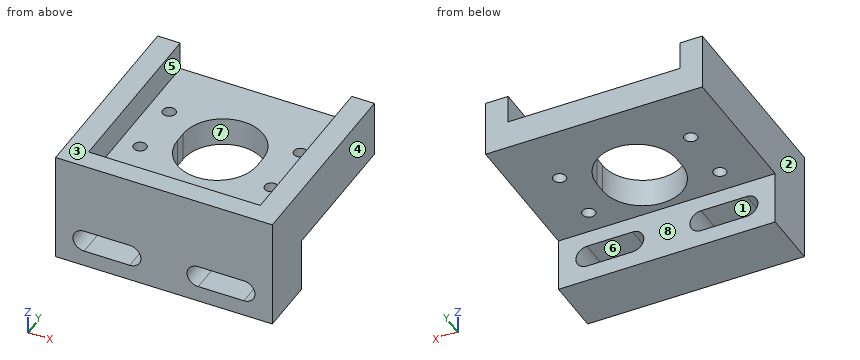
from build123d import *

# Parameters (mm, degrees)
SKETCH1_W                = 38
SKETCH1_H                = 19.5
BOSS_EXTRUDE1_DEPTH      = 35
SKETCH2_W                = 38
SKETCH2_H                = 9.5
CUT_EXTRUDE1_DEPTH       = 25
F_6_32_SLOT_REACH        = 12
APERTURE_THRU_HOLE_REACH = 21.5
SKETCH5_4_R              = 1.13
CUT_EXTRUDE5_DEPTH       = 5
F_4_40_TAPPED_HOLE1_D    = 2.2606


with BuildPart() as part:
    # Sketch1 → Boss-Extrude1 (new body)
    with BuildSketch(Plane(origin=(0, 0, 0), x_dir=(1, 0, 0), z_dir=(0, 1, 0))):
        with Locations((-7.223776224, 34.305944056)):
            Rectangle(SKETCH1_W, SKETCH1_H)
    extrude(amount=BOSS_EXTRUDE1_DEPTH)

    # Sketch2 → Cut-Extrude1 (cut)
    with BuildSketch(Plane(origin=(0, 35, 0), x_dir=(1, 0, 0), z_dir=(0, 1, 0))):
        with Locations((-7.223776224, 39.305944056)):
            Rectangle(SKETCH2_W, SKETCH2_H)
    extrude(amount=-CUT_EXTRUDE1_DEPTH, mode=Mode.SUBTRACT)

    # Sketch4 → 6-32 slot (cut, up to next)
    with BuildSketch(Plane(origin=(0, 10, 0), x_dir=(1, 0, 0), z_dir=(0, 1, 0)), mode=Mode.PRIVATE) as f_6_32_slot_sk1:
        with BuildLine():
            ThreePointArc((-13.223776224, 41.225951608), (-11.268776224, 39.270951608), (-13.223776224, 37.315951608))
            Line((-13.223776224, 37.315951608), (-21.223776224, 37.315951608))
            ThreePointArc((-21.223776224, 37.315951608), (-23.178776224, 39.270951608), (-21.223776224, 41.225951608))
            Line((-21.223776224, 41.225951608), (-13.223776224, 41.225951608))
        make_face()
    f_6_32_slot_tool1 = extrude(f_6_32_slot_sk1.sketch, amount=-F_6_32_SLOT_REACH, mode=Mode.PRIVATE) & part.part
    add(f_6_32_slot_tool1.solids().sort_by_distance((-17.223776, 10, -39.270952))[0], mode=Mode.SUBTRACT)
    # Sketch4 → 6-32 slot (cut, up to next)
    with BuildSketch(Plane(origin=(0, 10, 0), x_dir=(1, 0, 0), z_dir=(0, 1, 0)), mode=Mode.PRIVATE) as f_6_32_slot_sk2:
        with BuildLine():
            Line((6.776223776, 41.225951608), (-1.223776224, 41.225951608))
            ThreePointArc((-1.223776224, 41.225951608), (-3.178776224, 39.270951608), (-1.223776224, 37.315951608))
            Line((-1.223776224, 37.315951608), (6.776223776, 37.315951608))
            ThreePointArc((6.776223776, 37.315951608), (8.731223776, 39.270951608), (6.776223776, 41.225951608))
        make_face()
    f_6_32_slot_tool2 = extrude(f_6_32_slot_sk2.sketch, amount=-F_6_32_SLOT_REACH, mode=Mode.PRIVATE) & part.part
    add(f_6_32_slot_tool2.solids().sort_by_distance((2.776224, 10, -39.270952))[0], mode=Mode.SUBTRACT)

    # Sketch5 → aperture thru hole (cut, up to next)
    with BuildSketch(Plane.XY.offset(-24.555944056), mode=Mode.PRIVATE) as aperture_thru_hole_sk1:
        with BuildLine():
            Line((-14.223776224, 18.3), (-14.223776224, 20.3))
            ThreePointArc((-14.223776224, 20.3), (-7.223776224, 27.3), (-0.223776224, 20.3))
            Line((-0.223776224, 20.3), (-0.223776224, 18.3))
            ThreePointArc((-0.223776224, 18.3), (-7.223776224, 11.3), (-14.223776224, 18.3))
        make_face()
    aperture_thru_hole_tool1 = extrude(aperture_thru_hole_sk1.sketch, amount=-APERTURE_THRU_HOLE_REACH, mode=Mode.PRIVATE) & part.part
    add(aperture_thru_hole_tool1.solids().sort_by_distance((-7.223776, 19.3, -24.555944))[0], mode=Mode.SUBTRACT)

    # Sketch5<4> → Cut-Extrude5 (cut)
    with BuildSketch(Plane.XY.offset(-24.555944056)):
        with BuildLine():
            Line((-7.223776224, 27.3), (-7.223776224, 35))
            Line((-7.223776224, 35), (-22.273776224, 35))
            Line((-22.273776224, 35), (-22.273776224, 19.3))
            Line((-22.273776224, 19.3), (-14.223776224, 19.3))
            Line((-14.223776224, 19.3), (-14.223776224, 20.3))
            ThreePointArc((-14.223776224, 20.3), (-12.173523692, 25.249747468), (-7.223776224, 27.3))
        make_face()
        with Locations((-18.723776224, 24.3)):
            Circle(SKETCH5_4_R, mode=Mode.SUBTRACT)
        with BuildLine():
            Line((7.826223776, 35), (-7.223776224, 35))
            Line((-7.223776224, 35), (-7.223776224, 27.3))
            ThreePointArc((-7.223776224, 27.3), (-2.274028755, 25.249747468), (-0.223776224, 20.3))
            Line((-0.223776224, 20.3), (-0.223776224, 19.3))
            Line((-0.223776224, 19.3), (7.826223776, 19.3))
            Line((7.826223776, 19.3), (7.826223776, 35))
        make_face()
        with Locations((4.276223776, 24.3)):
            Circle(SKETCH5_4_R, mode=Mode.SUBTRACT)
        with BuildLine():
            Line((7.826223776, 3.6), (7.826223776, 19.3))
            Line((7.826223776, 19.3), (-0.223776224, 19.3))
            Line((-0.223776224, 19.3), (-0.223776224, 18.3))
            ThreePointArc((-0.223776224, 18.3), (-2.274028755, 13.350252532), (-7.223776224, 11.3))
            Line((-7.223776224, 11.3), (-7.223776224, 3.6))
            Line((-7.223776224, 3.6), (7.826223776, 3.6))
        make_face()
        with Locations((4.276223776, 14.3)):
            Circle(SKETCH5_4_R, mode=Mode.SUBTRACT)
        with BuildLine():
            Line((-14.223776224, 19.3), (-22.273776224, 19.3))
            Line((-22.273776224, 19.3), (-22.273776224, 3.6))
            Line((-22.273776224, 3.6), (-7.223776224, 3.6))
            Line((-7.223776224, 3.6), (-7.223776224, 11.3))
            ThreePointArc((-7.223776224, 11.3), (-12.173523692, 13.350252532), (-14.223776224, 18.3))
            Line((-14.223776224, 18.3), (-14.223776224, 19.3))
        make_face()
        with Locations((-18.723776224, 14.3)):
            Circle(SKETCH5_4_R, mode=Mode.SUBTRACT)
    extrude(amount=-CUT_EXTRUDE5_DEPTH, mode=Mode.SUBTRACT)

    # #4-40 Tapped Hole1 (through all)
    with Locations(Plane.XY.offset(-24.555944056)):
        with Locations((-18.723776224, 24.3), (-18.723776224, 14.3), (4.276223776, 14.3), (4.276223776, 24.3)):
            Hole(F_4_40_TAPPED_HOLE1_D / 2)


solid = part.part
Read the model definition and answer for the solid it produces. Units are mm, in the model's axes. Face numbers are marked on the shaded views. A direction names the side the tool comes from. Round coordinates to 2 decimals unless told otherwise and drop trailing zeros. Write each loop counter-clockwise with the first axis right and the second up, starting at its lowest first coordinate (ties: lowest second). Pieces come first, ordered by that corner, then holes. Notation, with made-up numbers: (73, 16) - (101, 16) arc R9 ccw to (101, 32) - close; hole circle Ø2 at (43.25, 19.25). An arc over 180 degrees is marked (long way). Use a Markdown table: item, result.
(1) The mould has two halves that part along X. Classify the marked faces 1, 2 and 3: released by +X, released by -X, zero draft, split by the parting line, or undercut.
Reported:
| item | result |
|---|---|
| face 1 | undercut |
| face 2 | released by -X |
| face 3 | zero draft |
(2) The part is cut by section C-C (y = 14.3). Write down the section's boundary in (x, z), then the cut area to 3 significant figures.
Reported:
| item | result |
|---|---|
| outline | (-26.22, -34.56) - (-19.85, -34.56) - (-19.85, -29.56) - (-22.27, -29.56) - (-22.27, -24.56) - (-26.22, -24.56) - close; (-17.59, -34.56) - (-12.97, -34.56) - (-12.97, -29.56) - (-17.59, -29.56) - close; (-1.48, -34.56) - (3.15, -34.56) - (3.15, -29.56) - (-1.48, -29.56) - close; (5.41, -34.56) - (11.78, -34.56) - (11.78, -24.56) - (7.83, -24.56) - (7.83, -29.56) - (5.41, -29.56) - close |
| area | 149 mm2 |
(3) Each of these flat-tipped pins is pushed along its axis until it touches: pin 1 Ø3 at (x, y) = (4.28, 14.3) entering from +Z; pin 2 Ø7.5 at (x, z) = (-15, -39) entering from +Y; pin 3 Ø6.5 at (x, y) = (-18.5, 6) entering from +Z; pin 4 Ø2 at (x, y) = (1, 28) entering from -Z. Where does it stop, or does it pass through?
Reported:
| item | result |
|---|---|
| pin 1 | z = -29.56 |
| pin 2 | y = 10 |
| pin 3 | z = -24.56 |
| pin 4 | z = -34.56 |
(4) The part is cut by section A-A (y = 21). Write down the section's boundary in (x, z).
Reported:
| item | result |
|---|---|
| outline | (-26.22, -34.56) - (-14.19, -34.56) - (-14.19, -29.56) - (-22.27, -29.56) - (-22.27, -24.56) - (-26.22, -24.56) - close; (-0.26, -34.56) - (11.78, -34.56) - (11.78, -24.56) - (7.83, -24.56) - (7.83, -29.56) - (-0.26, -29.56) - close |
(5) The part is cut by section B-B (z = -30.75). Write down the section's boundary in (x, y).
Reported:
| item | result |
|---|---|
| outline | (-26.22, 0) - (11.78, 0) - (11.78, 35) - (-26.22, 35) - close; hole circle Ø2.26 at (-18.72, 14.3); hole circle Ø2.26 at (-18.72, 24.3); hole (-14.22, 18.3) arc R7 ccw to (-0.22, 18.3) - (-0.22, 20.3) arc R7 ccw to (-14.22, 20.3) - close; hole circle Ø2.26 at (4.28, 14.3); hole circle Ø2.26 at (4.28, 24.3) |
(6) Straight lines are drawn through the part: line 1 along X through (y, z) = (26.5, -29.5); line 2 along Z through (x, y) = (-15, 2.5); line 3 along Y through (x, z) = (10, -42.25). For each, find the intervals that lie inside material, in ascending order. Write a range as [from, to].
Reported:
| item | result |
|---|---|
| line 1 | [-26.22, -22.27], [7.83, 11.78] |
| line 2 | [-44.06, -41.23], [-37.32, -24.56] |
| line 3 | [0, 10] |
(7) The part is cut by section D-D (z = -39.75). Write down the section's boundary in (x, y), then the cut area to 3 significant figures.
Reported:
| item | result |
|---|---|
| outline | (-26.22, 0) - (-23.12, 0) - (-23.12, 10) - (-26.22, 10) - close; (-11.33, 0) - (-3.12, 0) - (-3.12, 10) - (-11.33, 10) - close; (8.67, 0) - (11.78, 0) - (11.78, 10) - (8.67, 10) - close |
| area | 144 mm2 |
(8) Which of the six approach directions +Z, -Z, +X, -X, +Y, -Y give full straight-line access (tool end or side, diameter ignored) to the marked faces 4, 5, 6, 7 and 8?
Reported:
| item | result |
|---|---|
| face 4 | +Z, -Z, +X, +Y, -Y |
| face 5 | +Z, +Y |
| face 6 | +Y, -Y |
| face 7 | +Z, -Z |
| face 8 | -Z, +X, -X, +Y |
